```python
from build123d import *

# Parameters (mm, degrees)
F1_DEPTH = 39
F2_DEPTH = 35
F4_DEPTH = 33


with BuildPart() as f1:
    # F0 (on Top) → F1 (new body)
    with BuildSketch(Plane.XY):
        with BuildLine():
            ThreePointArc((55, -15), (52.0710678119, -7.9289321881), (45, -5))
            ThreePointArc((45, -5), (37.9289321881, -22.0710678119), (55, -15))
        make_face()
        with BuildLine():
            ThreePointArc((53, -15), (39.3431457505, -20.6568542495), (45, -7))
            ThreePointArc((45, -7), (50.6568542495, -9.3431457505), (53, -15))
        make_face(mode=Mode.SUBTRACT)
    extrude(amount=F1_DEPTH)



with BuildPart() as f1b:
    # F0 (on Top) → F1, piece 2 (new body)
    with BuildSketch(Plane.XY):
        with BuildLine():
            ThreePointArc((25, -15), (15, -5), (5, -15))
            ThreePointArc((5, -15), (15, -25), (25, -15))
        make_face()
        with BuildLine():
            ThreePointArc((23, -15), (15, -23), (7, -15))
            ThreePointArc((7, -15), (15, -7), (23, -15))
        make_face(mode=Mode.SUBTRACT)
    extrude(amount=F1_DEPTH)


with BuildPart() as f1c:
    # F0 (on Top) → F1, piece 3 (new body)
    with BuildSketch(Plane.XY):
        with BuildLine():
            ThreePointArc((25, -45), (7.9289321881, -37.9289321881), (15, -55))
            ThreePointArc((15, -55), (22.0710678119, -52.0710678119), (25, -45))
        make_face()
        with BuildLine():
            ThreePointArc((23, -45), (20.6568542495, -50.6568542495), (15, -53))
            ThreePointArc((15, -53), (9.3431457505, -39.3431457505), (23, -45))
        make_face(mode=Mode.SUBTRACT)
    extrude(amount=F1_DEPTH)


with BuildPart() as f1d:
    # F0 (on Top) → F1, piece 4 (new body)
    with BuildSketch(Plane.XY):
        with BuildLine():
            ThreePointArc((55, -45), (37.9289321881, -37.9289321881), (45, -55))
            ThreePointArc((45, -55), (52.0710678119, -52.0710678119), (55, -45))
        make_face()
        with BuildLine():
            ThreePointArc((53, -45), (50.6568542495, -50.6568542495), (45, -53))
            ThreePointArc((45, -53), (39.3431457505, -39.3431457505), (53, -45))
        make_face(mode=Mode.SUBTRACT)
    extrude(amount=F1_DEPTH)


with BuildPart() as f1_1:
    add(f1.part)

    add(f1b.part)  # F2 merges F1b

    add(f1c.part)  # F2 merges F1c

    add(f1d.part)  # F2 merges F1d
    # F0 (on Top) → F2 (join)
    with BuildSketch(Plane.XY):
        Polygon((15, 0), (0, 0), (0, -15), (0, -45), (0, -60), (15, -60), (45, -60), (60, -60), (60, -45), (60, -8.6315972731), (60, 0), (45, 0), align=None)
        with BuildLine():
            ThreePointArc((25, -45), (22.0710678119, -52.0710678119), (15, -55))
            ThreePointArc((15, -55), (7.9289321881, -37.9289321881), (25, -45))
        make_face(mode=Mode.SUBTRACT)
        with BuildLine():
            ThreePointArc((55, -45), (52.0710678119, -52.0710678119), (45, -55))
            ThreePointArc((45, -55), (37.9289321881, -37.9289321881), (55, -45))
        make_face(mode=Mode.SUBTRACT)
        with BuildLine():
            ThreePointArc((25, -15), (15, -25), (5, -15))
            ThreePointArc((5, -15), (15, -5), (25, -15))
        make_face(mode=Mode.SUBTRACT)
        with BuildLine():
            ThreePointArc((55, -15), (37.9289321881, -22.0710678119), (45, -5))
            ThreePointArc((45, -5), (52.0710678119, -7.9289321881), (55, -15))
        make_face(mode=Mode.SUBTRACT)
    extrude(amount=F2_DEPTH)

    # F3 (on Top) → F4 (cut)
    with BuildSketch(Plane.XY):
        Polygon((2, -30), (2, -58), (58, -58), (58, -2), (2, -2), align=None)
    extrude(amount=F4_DEPTH, mode=Mode.SUBTRACT)


solid = f1_1.part
```
The listing builds one solid part. Answer for the finished solid, in the listing's coordinates (mm). A direction names the side the tool comes from. Coordinates: 2 decimals unless noted, no trailing zeros. Loops run counter-clockwise (first coordinate to the right, second up) from the corner with the lowest first, then second, coordinate; pieces in that order, holes last. Notation, with made-up numbers: M -30.5,82.25 L 19.5,82.25 A16 ccw 19.5,88.25 Z; hole C 54.5,63.5 d4. An arc over 180 degrees is marked long. Answer as a JSON object with one key per item and string values. Group by question number.
Item 1: Section A-A (y = -21.5) is taken. Write down the section's boundary in (x, z), and give its area (3 significant figures).
Item 2: Consider L1, parallel to Y at x = 15, z = 36; L2, parallel to Y at x = 15, z = 34.65; L3, parallel to Y at x = 29.5, z = 7. Determine where each line is inside the solid, lowest interval first.
Item 3: Determine the mould class of faces 1 (the face through (5.46, -18, 36.97)), 2 (the face through (60, -30, 17)), 3 (the face through (15, -6.8, 39)) for opening direction X: +X half, -X half, draft (parallel to the pull), parting line (faces both ways), or undercut.
Item 4: Section C-C (x = 27.5) is taken. Write down the section's boundary in (y, z).
Item 5: Section D-D (z = 23.5) is taken. Write down the section's boundary in (x, y), and give its area (3 significant figures).
Item 6: Section B-B (x = 48) is taken. Write down the section's boundary in (y, z).
Item 7: Which of the six approach directions +Z, -Z, +X, -X, +Y, -Y give full straight-line access (tool end or side, diameter ignored) to faces 4 (the face through (30, -30, 35)), 5 (the face through (30, -30, 33)), 6 (the face through (45, -6.8, 39))?
Item 8: Each of these flat-tipped pins is pushed along its axis until it touches: P1, Ø10, axis at y = -20, z = 9.5, coming from the -X side; P2, Ø18.5, axis at x = 15, y = -45, coming from the -Z side; P3, Ø4, axis at x = 15.5, y = -40.5, coming from the +Z side. Where does it stop, or does it pass through?
Solved:
{
 "1": {"outline": "M 0,0 L 2,0 L 2,33 L 10.34,33 L 10.34,39 L 7.4,39 L 7.4,35 L 0,35 Z; M 19.66,33 L 40.34,33 L 40.34,39 L 37.4,39 L 37.4,35 L 22.6,35 L 22.6,39 L 19.66,39 Z; M 49.66,33 L 58,33 L 58,0 L 60,0 L 60,35 L 52.6,35 L 52.6,39 L 49.66,39 Z", "area": "262 mm2"},
 "2": {"L1": "y = -55 to -53, -37 to -35, -25 to -23, -7 to -5", "L2": "y = -60 to -53, -37 to -23, -7 to 0", "L3": "y = -60 to -58, -2 to 0"},
 "3": {"face 1": "undercut", "face 2": "+X half", "face 3": "draft"},
 "4": {"outline": "M -60,0 L -58,0 L -58,33 L -2,33 L -2,0 L 0,0 L 0,35 L -60,35 Z"},
 "5": {"outline": "M 0,-60 L 60,-60 L 60,0 L 0,0 Z; hole M 2,-58 L 58,-58 L 58,-2 L 2,-2 Z", "area": "464 mm2"},
 "6": {"outline": "M -60,0 L -58,0 L -58,33 L -52.42,33 L -52.42,39 L -54.54,39 L -54.54,35 L -60,35 Z; M -37.58,33 L -22.42,33 L -22.42,39 L -24.54,39 L -24.54,35 L -35.46,35 L -35.46,39 L -37.58,39 Z; M -7.58,33 L -2,33 L -2,0 L 0,0 L 0,35 L -5.46,35 L -5.46,39 L -7.58,39 Z"},
 "7": {"face 4": "+Z", "face 5": "-Z", "face 6": "+Z, +X, -X, +Y, -Y"},
 "8": {"P1": "stops at x = 0", "P2": "stops at z = 33", "P3": "passes through"}
}
